from build123d import *

# Parameters (mm, degrees)
BOSS_EXTRUDE1_DEPTH = 64
SKETCH2_R           = 2.499999953
CUT_EXTRUDE2_DEPTH  = 5
SKETCH3_W           = 8
SKETCH3_H           = 13
SKETCH3_H_2         = 12
CUT_EXTRUDE3_DEPTH  = 15


with BuildPart() as part:
    # Sketch1 → Boss-Extrude1 (new body)
    with BuildSketch(Plane.XY):
        with BuildLine():
            Line((0, 0), (21.499999926, 0))
            Line((21.499999926, 0), (21.499999926, 1.4))
            Line((21.499999926, 1.4), (2.799999992, 1.4))
            ThreePointArc((2.799999992, 1.4), (-1.565247581, 6.630495138), (0, 0))
        make_face()
    extrude(amount=BOSS_EXTRUDE1_DEPTH)

    # Sketch2 → Cut-Extrude2 (cut)
    with BuildSketch(Plane(origin=(0, 0, 0), x_dir=(1, 0, 0), z_dir=(0, 1, 0))):
        with Locations(Location((11.999999876, -53.99999995, 0), (0, 0, 90))):
            Circle(SKETCH2_R)
        with Locations(Location((13.999999876, -32.000000008, 0), (0, 0, 90))):
            Circle(SKETCH2_R)
        with Locations(Location((11.999999876, -10.000000066, 0), (0, 0, 90))):
            Circle(SKETCH2_R)
    extrude(amount=CUT_EXTRUDE2_DEPTH, mode=Mode.SUBTRACT)

    # Sketch3 → Cut-Extrude3 (cut)
    with BuildSketch(Plane(origin=(0, 0, 0), x_dir=(1, 0, 0), z_dir=(0, 1, 0))):
        with Locations((0, -6.5)):
            Rectangle(SKETCH3_W, SKETCH3_H)
        with Locations((0, -32)):
            Rectangle(SKETCH3_W, SKETCH3_H_2)
        with Locations((0, -57.5)):
            Rectangle(SKETCH3_W, SKETCH3_H)
    extrude(amount=CUT_EXTRUDE3_DEPTH, mode=Mode.SUBTRACT)


solid = part.part
The model under review builds one solid part; all positions refer to its coordinate system, in mm. A direction names the side the tool comes from. Round coordinates to 2 decimals unless told otherwise and drop trailing zeros. Write each loop counter-clockwise with the first axis right and the second up, starting at its lowest first coordinate (ties: lowest second). Pieces come first, ordered by that corner, then holes. Notation, with made-up numbers: M 38.5,-4.75 L 49.5,-4.75 A19 ccw 49.5,15.25 Z; hole C 85.5,33.25 d8. An arc over 180 degrees is marked long. Answer as CSV lines item,"result". Start each with the question number.
Q1. Consider section D-D, the plane z = 15. Give the boundary of the cut face in (x, y), then the cut area to 3 significant figures.
Q2. Consider section C-C, the plane x = 10.75. Give the boundary of the cut face in (y, z).
Q3. Consider section B-B, the plane y = 5.5. Give the boundary of the cut face in (x, z).
Q4. The part is to be moulded in two halves that separate along Z. For faces 5 (the face through (0, 3, 26)), 6 (the face through (13, 1, 0)), 7 (the face through (4, 1, 7)), say which applies: +Z half, -Z half, draft (parallel to the pull), parting line (faces both ways), or undercut.
Q5. Consider section A-A, the plane z = 54. Give the boundary of the cut face in (x, y).
Q6. Tool access review of faces 1 (the face through (0, 3, 13)), 2 (the face through (13.5, 0.7, 56)), 3 (the face through (0, 3, 38)), 4 (the face through (0, 3, 51)): name each direction out of +Z, -Z, +X, -X, +Y, -Y from which nothing blocks a thin tool from reaching the whole face with its end or side.
Q7. Wall thickness on line 1 along X through (y, z) = (0.65, 54); line 2 along Z through (x, y) = (14, 0.75); line 3 along Z through (x, y) = (12, 1): over which ranges is each line inside the solid? List them lowest first.
Q8. Clearance check with flat-ended pins moving along their axes: P1, Ø2, axis at x = 1.5, y = 2.5, coming from the -Z side; P2, Ø5.5, axis at x = 8.5, z = 33.5, coming from the +Y side; P3, Ø0.7, axis at y = 0.5, z = 34, coming from the -X side. State where each tip first meets the part, or that it passes through.
Result set:
1,outline,"M 0,0 L 21.5,0 L 21.5,1.4 L 2.8,1.4 A3.5 ccw long Z"
1,area,"65.8 mm²"
2,outline,"M 0,0 L 1.4,0 L 1.4,7.83 L 0,7.83 Z; M 0,12.17 L 1.4,12.17 L 1.4,51.83 L 0,51.83 Z; M 0,56.17 L 1.4,56.17 L 1.4,64 L 0,64 Z"
3,outline,"M -2.87,13 L 2.87,13 L 2.87,26 L -2.87,26 Z; M -2.87,38 L 2.87,38 L 2.87,51 L -2.87,51 Z"
4,face 5,"undercut"
4,face 6,"-Z half"
4,face 7,"draft"
5,outline,"M 4,0 L 9.5,0 L 9.5,1.4 L 4,1.4 Z; M 14.5,0 L 21.5,0 L 21.5,1.4 L 14.5,1.4 Z"
6,face 1,"-Z, -X, +Y, -Y"
6,face 2,"+Y, -Y"
6,face 3,"-X, +Y, -Y"
6,face 4,"+Z, -X, +Y, -Y"
7,line 1,"x = 4 to 9.5, 14.5 to 21.5"
7,line 2,"z = 0 to 8.5, 11.5 to 29.5, 34.5 to 52.5, 55.5 to 64"
7,line 3,"z = 0 to 7.5, 12.5 to 30.5, 33.5 to 51.5, 56.5 to 64"
8,P1,"stops at z = 13"
8,P2,"stops at y = 1.4"
8,P3,"stops at x = 4"
